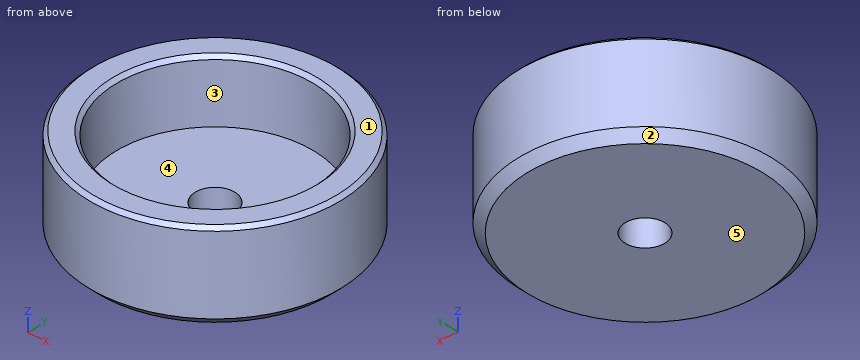
from build123d import *

# Parameters (mm, degrees)
F0_R     = 70
F1_DEPTH = 50
F2_R     = 55
F3_DEPTH = 35
F4_SIZE  = 5
F5_SIZE  = 2
F7_D     = 22
F7_DEPTH = 30
F7_TIP   = 6.6094668093


with BuildPart() as f1:
    # F0 (on Top) → F1 (new body)
    with BuildSketch(Plane.XY):
        Circle(F0_R)
    extrude(amount=F1_DEPTH)

    # F2 (on face) → F3 (cut)
    with BuildSketch(Plane.XY.offset(50)):
        Circle(F2_R)
    extrude(amount=-F3_DEPTH, mode=Mode.SUBTRACT)

    # F4
    f4_edges = [f1.edges().sort_by_distance(p)[0] for p in [
        (-70, 0, 0),
    ]]
    chamfer(f4_edges, length=F4_SIZE)

    # F5
    f5_edges = [f1.edges().sort_by_distance(p)[0] for p in [
        (-70, 0, 50),
        (-55, 0, 50),
    ]]
    chamfer(f5_edges, length=F5_SIZE)

    # F7
    with Locations(Plane(origin=(0, 0, 0), x_dir=(1, 0, 0), z_dir=(0, 0, -1))):
        with Locations((0, 0)):
            Hole(F7_D / 2, depth=F7_DEPTH)
            with Locations((0, 0, -(F7_DEPTH + F7_TIP / 2))):  # 118° drill point
                Cone(0, F7_D / 2, F7_TIP, mode=Mode.SUBTRACT)


solid = f1.part
Part model, mm, in its own coordinate system. Face numbers are marked on the shaded views. A direction names the side the tool comes from. Coordinates: 2 decimals unless noted, no trailing zeros. Loops run counter-clockwise (first coordinate to the right, second up) from the corner with the lowest first, then second, coordinate; pieces in that order, holes last. Notation, with made-up numbers: (59, 88) - (89, 88) arc R27 ccw to (89, 121) - close; hole circle Ø5 at (16.5, 2). An arc over 180 degrees is marked (long way). Write each question's results on one line, items separated by ' | '. Start each with the question number.
Q1. Two-plate mould, pull along Y, no slides. Class the marked faces 1, 2 and 3: +Y half, -Y half, draft (parallel to the pull), parting line (faces both ways), or undercut.
Q2. Slice it at C-C on z = 39.5. Give the cut face in (x, y).
Q3. Slice it at A-A on y = 0. Give the cut face in (x, z).
Q4. Probe line 1 along Y through (x, z) = (0, 34); line 2 along Y through (x, z) = (0, 7.5); line 3 along Z through (x, y) = (28, -16). List the from-to ranges inside material, lowest first.
Q5. Slice it at D-D on z = 9. Give the cut face in (x, y), and give its area (3 significant figures).
Q6. Which spindle directions (+Z, -Z, +X, -X, +Y, -Y) get a long thin tool onto all of the face, cutting with end or side? Do the marked faces 4 and 5. Say none if no direction does.
Q7. Drop flat-ended pins along their axis: pin 1 Ø2 at (x, y) = (12.5, 18) entering from -Z; pin 2 Ø1 at (x, z) = (39.5, 20.5) entering from -Y; pin 3 Ø6 at (y, z) = (27.5, 26.5) entering from +X; pin 4 Ø12 at (y, z) = (36, 16.5) entering from +X. Give the stop position or say it passes through.
Answer:
1) face 1: draft | face 2: parting line | face 3: undercut
2) outline: circle Ø140 at (0, 0); hole circle Ø110 at (0, 0)
3) outline: (-70, 5) - (-65, 0) - (-11, 0) - (-11, 15) - (-55, 15) - (-55, 48) - (-57, 50) - (-68, 50) - (-70, 48) - close; (11, 0) - (65, 0) - (70, 5) - (70, 48) - (68, 50) - (57, 50) - (55, 48) - (55, 15) - (11, 15) - close
4) line 1: y = -70 to -55, 55 to 70 | line 2: y = -70 to -11, 11 to 70 | line 3: z = 0 to 15
5) outline: circle Ø140 at (0, 0); hole circle Ø22 at (0, 0) | area: 15,000 mm2
6) face 4: +Z | face 5: -Z, +X, -X, +Y, -Y
7) pin 1: stops at z = 0 | pin 2: stops at y = -58.13 | pin 3: stops at x = 65.57 | pin 4: stops at x = 63.25
